The model under review builds one solid part; all positions refer to its coordinate system, in mm. A direction names the side the tool comes from. Round coordinates to 2 decimals unless told otherwise and drop trailing zeros. Write each loop counter-clockwise with the first axis right and the second up, starting at its lowest first coordinate (ties: lowest second). Pieces come first, ordered by that corner, then holes. Notation, with made-up numbers: (89, 70.25) - (117, 70.25) arc R34 cw to (117, 106.25) - close; hole circle Ø6 at (65.25, 34). An arc over 180 degrees is marked (long way). Return JSON: item names as keys, results as strings.
from build123d import *

# Parameters (mm, degrees)
BASE_FLANGE1_DEPTH = 10
CUT_EXTRUDE1_REACH = 155.346
SKETCH7_R          = 2.5


# Sheet-metal steps are written as plain solids
with BuildPart() as part:
    # Sketch2 → Base-Flange1 (new body)
    with BuildSketch(Plane.XY):
        with BuildLine():
            Line((7.5, 49.434299833), (7.5, 144.62))
            Line((7.5, 144.62), (-7.5, 144.62))
            Line((-7.5, 144.62), (-7.5, 49.434299833))
            ThreePointArc((-7.5, 49.434299833), (0, -50), (7.5, 49.434299833))
        make_face()
    extrude(amount=-BASE_FLANGE1_DEPTH)

    # Sketch7 → Cut-Extrude1 (cut, up to next)
    with BuildSketch(Plane.XY, mode=Mode.PRIVATE) as cut_extrude1_sk1:
        with Locations((0, 134.62)):
            Circle(SKETCH7_R)
    cut_extrude1_tool1 = extrude(cut_extrude1_sk1.sketch, amount=-CUT_EXTRUDE1_REACH, mode=Mode.PRIVATE) & part.part
    # Sketch7 → Cut-Extrude1 (cut, up to next)
    with BuildSketch(Plane.XY, mode=Mode.PRIVATE) as cut_extrude1_sk2:
        Circle(SKETCH7_R)
    cut_extrude1_tool2 = extrude(cut_extrude1_sk2.sketch, amount=-CUT_EXTRUDE1_REACH, mode=Mode.PRIVATE) & part.part
    add(cut_extrude1_tool1.solids().sort_by_distance((0, 134.62, 0))[0], mode=Mode.SUBTRACT)
    add(cut_extrude1_tool2.solids().sort_by_distance((0, 0, 0))[0], mode=Mode.SUBTRACT)


solid = part.part
(1) Wall thickness on line 1 (X direction, y = 134.62, z = -6); line 2 (X direction, y = 118.5, z = -8); line 3 (Y direction, x = 43.5, z = -8.75): over which ranges is each line inside the solid? List them lowest first.
Filled in:
{"line 1": "x = -7.5 to -2.5, 2.5 to 7.5", "line 2": "x = -7.5 to 7.5", "line 3": "y = -24.65 to 24.65"}
(2) Add section D-D (y = 0). Write out the cut boundary in (x, z), plus the area to 3 significant figures.
Filled in:
{"outline": "(-50, -10) - (-2.5, -10) - (-2.5, 0) - (-50, 0) - close; (2.5, -10) - (50, -10) - (50, 0) - (2.5, 0) - close", "area": "950 mm2"}
(3) Add section C-C (x = 0). Write out the cut boundary in (y, z).
Filled in:
{"outline": "(-50, -10) - (-2.5, -10) - (-2.5, 0) - (-50, 0) - close; (2.5, -10) - (132.12, -10) - (132.12, 0) - (2.5, 0) - close; (137.12, -10) - (144.62, -10) - (144.62, 0) - (137.12, 0) - close"}
(4) Add section B-B (z = -4.25). Write out the cut boundary in (x, y).
Filled in:
{"outline": "(-7.5, 49.43) arc R50 ccw (long way) to (7.5, 49.43) - (7.5, 144.62) - (-7.5, 144.62) - close; hole circle Ø5 at (0, 0); hole circle Ø5 at (0, 134.62)"}
(5) Clearance check with flat-ended pins moving along their axes: pin 1 Ø6.5 at (x, y) = (0, 134.62) entering from -Z; pin 2 Ø3 at (x, z) = (31, -8.5) entering from -Y; pin 3 Ø5 at (y, z) = (112.5, -6.5) entering from +X; pin 4 Ø5 at (y, z) = (95.5, -7) entering from -X. State where each tip first meets the part, or that it passes through.
Filled in:
{"pin 1": "stops at z = -10", "pin 2": "stops at y = -40.37", "pin 3": "stops at x = 7.5", "pin 4": "stops at x = -7.5"}
(6) For faces 4 (the flat face through (7.5, 96, -5)), 5 (the flat face through (0, 144.62, -5)), list the 3-axis set-ups (+Z, -Z, +X, -X, +Y, -Y) from which the entire face can be reached by the end or side of a thin tool; tool diameter is ignored.
Filled in:
{"face 4": "+Z, -Z, +X, +Y", "face 5": "+Z, -Z, +X, -X, +Y"}
(7) Add section A-A (y = 134.62). Write out the cut boundary in (x, z), plus the area to 3 significant figures.
Filled in:
{"outline": "(-7.5, -10) - (-2.5, -10) - (-2.5, 0) - (-7.5, 0) - close; (2.5, -10) - (7.5, -10) - (7.5, 0) - (2.5, 0) - close", "area": "100 mm2"}
(8) Mouldability with a two-part tool opening along Y and no side actions: class faces 1 (the flat face through (-7.5, 98, -5)), 2 (the cylindrical face through (-2.093, -49.956, -4.93)), 3 (the cylindrical face through (-0.54, -2.44, -4.93)) as released by +Y, released by -Y, zero draft, split by the parting line, or undercut.
Filled in:
{"face 1": "zero draft", "face 2": "split by the parting line", "face 3": "undercut"}
